Autodesk Fusion 360 part; units mm, degrees
sketch "Sketch1" plane through (0, 0, 0) normal (0, 1, 0) x (1, 0, 0)
  circle A0 centre (150, 0) radius 4.95
  circle A1 centre (150, 0) radius 2.575
  dimension "d1" = 9.9
  dimension "d2" = 5.15
extrude "Extrude1" add sketch "Sketch1" along normal blind 13.15
ref_plane "WorkPlane1" through (150, 7.9424, 4.95) normal (0, 0, 1) x (-1, 0, 0)
sketch "Sketch2" plane through (0, 0, 4.95) normal (0, 0, 1) x (1, 0, 0)
  line L0 (154.95, 13.15) -> (145.05, 13.15) construction
  line L1 (154.95, 0) -> (145.05, 0) construction
  line L2 (150, 13.15) -> (150, 0) construction
  circle A0 centre (150, 8.15) radius 1.6
  dimension "d6" = 3.2
  dimension "d7" = 5
extrude "Extrude2" cut sketch "Sketch2" against normal blind 16
fillet "Fillet1" radius 1 2 edges at (145.385, 13.15, 1.79) (145.385, 0, 1.79)
Could you check a few things on this model? Use its own coordinates, in mm. Give positions to 0.01 mm unless a question says otherwise; leave off trailing zeros. Order: outer loops, then holes, each group sorted by start corner. A loop starts at its lowest first (then second) coordinate and runs counter-clockwise, first axis right, second up. Notation, with made-up numbers: (-23, 23) - (30, 23) arc R17 ccw to (30, 45) - close; hole circle Ø4 at (-4, 0.5). An arc over 180 degrees is marked (long way). One line per item, written item: value. Start each with the question number.
1. Imagine slicing it at A-A on y = 8.15. List the corners of the cut face in (x, z) for me (3 decimals).
2. If I drill on probe 1 along X at (y, z) = (4.25, 0) (3 decimals); probe 2 along Y at (x, z) = (150, -2.8); probe 3 along Z at (x, y) = (150, 4.75) (3 decimals), over which ranges is the centre line in solid material (lowest first)?
3. For P1, Ø3, axis at x = 150, y = 8.15, coming from the -Z side; P2, Ø4, axis at x = 146, y = 4.5, coming from the +Z side, each with a flat end and sliding along its axis, tell me the tip position at first contact or that it passes through.
4. Thinking about a two-plate mould opening in X: for faces 1 (the face through (150, 13.15, 3)), 2 (the face through (154.72, 6.5, 1.49)), 3 (the face through (147.427, 6.483, 0.113)), which applies, +X half, -X half, draft (parallel to the pull), parting line (faces both ways), or undercut?
5. Imagine slicing it at B-B on x = 150.5. Give the number of separate pieces and of enclosed holes in the cut face, plus the area to 3 significant figures.
6. Imagine slicing it at C-C on y = 3.25. List the corners of the cut face in (x, z) for me (3 decimals).
Values:
1. outline: (148.4, -4.684) - (148.4, -2.018) arc R2.575 cw to (148.4, 2.018) - (148.4, 4.684) arc R4.95 ccw to start; (151.6, -4.684) arc R4.95 ccw to (151.6, 4.684) - (151.6, 2.018) arc R2.575 cw to (151.6, -2.018) - close
2. probe 1: 145.05 to 147.425, 152.575 to 154.95
2. probe 2: 0 to 6.55, 9.75 to 13.15
2. probe 3: -4.95 to -2.575, 2.575 to 4.95
3. P1: through
3. P2: z = 4.53
4. face 1: draft
4. face 2: parting line
4. face 3: undercut
5. separate pieces: 4
5. enclosed holes: 0
5. area: 47.6 mm²
6. outline: circle Ø9.9 at (150, 0); hole circle Ø5.15 at (150, 0)
